Design review of the part shown in the three views and the two pictorial views. Dimensions are in mm from the part's minimum x, y and z. A direction names the side the tool comes from. Coordinates: 2 decimals unless noted, no trailing zeros. Write each loop counter-clockwise with the first axis right and the second up, starting at its lowest first coordinate (ties: lowest second). Pieces come first, ordered by that corner, then holes. Notation, with made-up numbers: (8.5, 45) -> (28.5, 45) arc R25 cw to (28.5, 57) -> close; hole circle Ø8 at (-12, 58). An arc over 180 degrees is marked (long way). Write item = value, one per line. Start each with the question number.
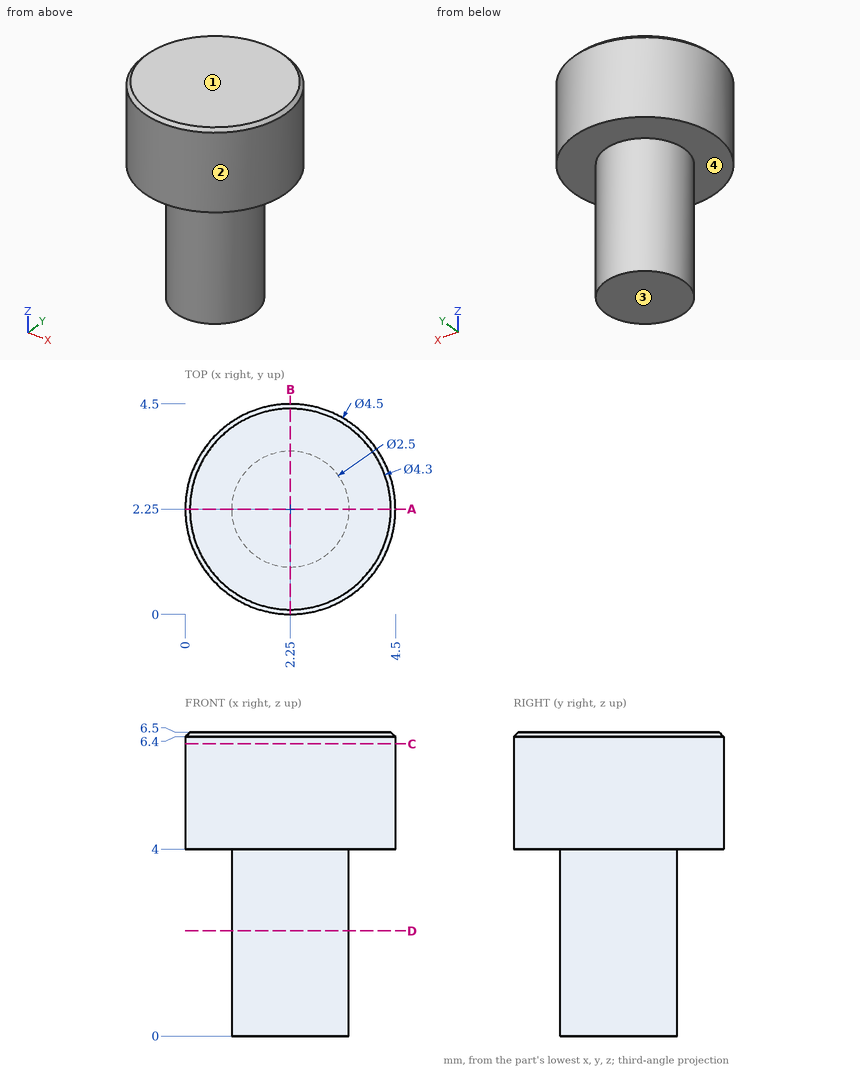
(1) Take a section at D-D, the plane z = 2.25. State the section outline as (x, y) points, then the cut area to 3 significant figures.
(2) Mouldability with a two-part tool opening along X and no side actions: class the marked faces 1 and 2 as pulls with the +X half, pulls with the -X half, needs draft (parallel to the pull), parting line crosses it, or undercut.
(3) Take a section at C-C, the plane z = 6.25. State the section outline as (x, y) points, then the cut area to 3 significant figures.
(4) For line 1 (Y direction, x = 2.35, z = 5); line 2 (Z direction, x = 4.1, y = 1.95); line 3 (X direction, y = 2.55, z = 3.5), list the stretches that pass through material, from the lowest coordinate up.
(5) For the marked faces 3 and 4, list the 3-axis set-ups (+Z, -Z, +X, -X, +Y, -Y) from which the entire face can be reached by the end or side of a thin tool; tool diameter is ignored.
(6) Take a section at A-A, the plane y = 2.25. State the section outline as (x, z) points, then the cut area to 3 significant figures.
Report:
q1.outline = circle Ø2.5 at (2.25, 2.25)
q1.area = 4.91 mm2
q2.face_1 = needs draft
q2.face_2 = parting line crosses it
q3.outline = circle Ø4.5 at (2.25, 2.25)
q3.area = 15.9 mm2
q4.line_1 = 0 to 4.5
q4.line_2 = 4 to 6.5
q4.line_3 = 1.04 to 3.46
q5.face_3 = -Z, +X, -X, +Y, -Y
q5.face_4 = -Z
q6.outline = (0, 4) -> (1, 4) -> (1, 0) -> (3.5, 0) -> (3.5, 4) -> (4.5, 4) -> (4.5, 6.4) -> (4.4, 6.5) -> (0.1, 6.5) -> (0, 6.4) -> close
q6.area = 21.2 mm2
